Geometry: final body of the model. Coordinates: model frame, mm. Round coordinates to 2 decimals unless told otherwise and drop trailing zeros. Order: outer loops, then holes, each group sorted by start corner. A loop starts at its lowest first (then second) coordinate and runs counter-clockwise, first axis right, second up. Notation, with made-up numbers: M -14.5,16.5 L -10.5,16.5 A17 cw -10.5,43.5 Z; hole C 24.5,88.25 d3. An arc over 180 degrees is marked long. Return JSON: item names as keys, results as strings. Group by question number.
Q1. Mould query, pull axis X, two halves, no side actions, for faces 1 (the face through (-3, -250, 14)), 2 (the face through (250, -3, 10)), 3 (the face through (-3, 4, 10)), 4 (the face through (-250, -3, 10)). Classes: released by +X, released by -X, zero draft, split by the parting line, or undercut.
Q2. Ray query, probe 1 along Y at (x, z) = (-200, 13.5); probe 2 along X at (y, z) = (-89, 2.75); probe 3 along Z at (x, y) = (229.5, -113). Return the intervals inside material, ascending.
Q3. Cut plane A-A on y = 43.5. Output: boundary loops of the cut face in (x, z).
Q4. Contact query for flat-ended pins moving along their axis: pin 1 (10 mm diameter, centred on x = -156, z = 3, fed in from -Y); pin 2 (4 mm diameter, centred on x = -168, y = -191, fed in from -Z). Output: stop coordinate, or through.
Q5. Cut plane B-B on x = -145. Output: boundary loops of the cut face in (y, z), and give its area (3 significant figures).
```python
from build123d import *

# Parameters (mm, degrees)
SKETCH1_W           = 500
SKETCH1_H           = 500
BOSS_EXTRUDE1_DEPTH = 20
SKETCH2_W           = 480
SKETCH2_H           = 10
CUT_EXTRUDE1_DEPTH  = 500
SKETCH3_R           = 5
CUT_EXTRUDE2_DEPTH  = 10


with BuildPart() as part:
    # Sketch1 → Boss-Extrude1 (new body)
    with BuildSketch(Plane.XY):
        Rectangle(SKETCH1_W, SKETCH1_H)
    extrude(amount=BOSS_EXTRUDE1_DEPTH)

    # Sketch2 → Cut-Extrude1 (cut)
    with BuildSketch(Plane(origin=(0, 250, 0), x_dir=(1, 0, 0), z_dir=(0, 1, 0))):
        with Locations((0, -5)):
            Rectangle(SKETCH2_W, SKETCH2_H)
    extrude(amount=-CUT_EXTRUDE1_DEPTH, mode=Mode.SUBTRACT)

    # Sketch3 → Cut-Extrude2 (cut)
    with BuildSketch(Plane.XY.offset(20)):
        with Locations((-200, 200)):
            Circle(SKETCH3_R)
        with Locations((200, 200)):
            Circle(SKETCH3_R)
        with Locations((-200, -200)):
            Circle(SKETCH3_R)
        with Locations((200, -200)):
            Circle(SKETCH3_R)
    extrude(amount=-CUT_EXTRUDE2_DEPTH, mode=Mode.SUBTRACT)


solid = part.part
```
Result sheet:
{
 "1": {"face 1": "zero draft", "face 2": "released by +X", "face 3": "undercut", "face 4": "released by -X"},
 "2": {"probe 1": "y = -250 to -205, -195 to 195, 205 to 250", "probe 2": "x = -250 to -240, 240 to 250", "probe 3": "z = 10 to 20"},
 "3": {"outline": "M -250,0 L -240,0 L -240,10 L 240,10 L 240,0 L 250,0 L 250,20 L -250,20 Z"},
 "4": {"pin 1": "passes through", "pin 2": "stops at z = 10"},
 "5": {"outline": "M -250,10 L 250,10 L 250,20 L -250,20 Z", "area": "5,000 mm²"}
}
